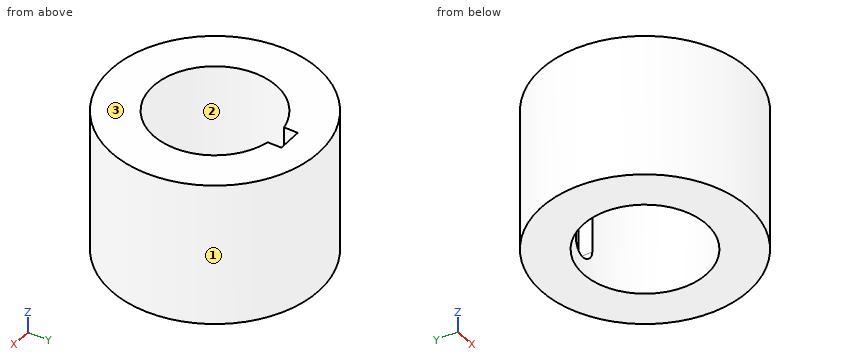
```python
from build123d import *

# Parameters (mm, degrees)
SKETCH1_R           = 21
SKETCH1_R_2         = 12.5
BOSS_EXTRUDE4_DEPTH = 29
SKETCH3_W           = 5
SKETCH3_H           = 5
CUT_EXTRUDE3_DEPTH  = 25.5
FILLET5_R           = 2.5
FILLET6_R           = 2.5


with BuildPart() as part:
    # Sketch1 → Boss-Extrude4 (new body)
    with BuildSketch(Plane.XY):
        with Locations(Location((0, 0, 0), (0, 0, 180))):
            Circle(SKETCH1_R)
        with Locations(Location((0, 0, 0), (0, 0, 180))):
            Circle(SKETCH1_R_2, mode=Mode.SUBTRACT)
    extrude(amount=BOSS_EXTRUDE4_DEPTH)

    # Sketch3 → Cut-Extrude3 (cut)
    with BuildSketch(Plane.XY.offset(29)):
        with Locations((0, 12.5)):
            Rectangle(SKETCH3_W, SKETCH3_H)
    extrude(amount=-CUT_EXTRUDE3_DEPTH, mode=Mode.SUBTRACT)

    # Fillet5
    fillet5_edges = [part.edges().sort_by_distance(p)[0] for p in [
        (2.5, 13.623724357, 3.5),
    ]]
    fillet(fillet5_edges, radius=FILLET5_R)

    # Fillet6
    fillet6_edges = [part.edges().sort_by_distance(p)[0] for p in [
        (-2.5, 13.623724357, 3.5),
    ]]
    fillet(fillet6_edges, radius=FILLET6_R - 0.0001)  # a hair under: the kernel refuses the full size


solid = part.part
```
Can you work these out from the model? Positions are in its coordinate system, mm. Face numbers are marked on the shaded views. Round coordinates to 2 decimals unless told otherwise and drop trailing zeros. Loops run counter-clockwise (first coordinate to the right, second up) from the corner with the lowest first, then second, coordinate; pieces in that order, holes last. Notation, with made-up numbers: (66, -15) -> (107, -15) arc R19 ccw to (107, 21) -> close; hole circle Ø1 at (4, -21). An arc over 180 degrees is marked (long way). One line per item, written item: value. Start each with the question number.
1. If I drill on probe 1 along Y at (x, z) = (0, 22.75); probe 2 along X at (y, z) = (10.5, 7); probe 3 along Y at (x, z) = (4, 26.25), over which ranges is the centre line in solid material (lowest first)?
2. If we section it at D-D, the plane y = -18: Write out the boundary of the cut face in (x, z).
3. If we mould it in two halves opening along X, with no side actions, what happens to the marked faces 1, 2 and 3? For each: pulls with the +X half, pulls with the -X half, needs draft (parallel to the pull), parting line crosses it, or undercut.
4. For pin 1 (1 mm diameter, centred on x = -13.5, z = 6, fed in from +Y); pin 2 (0.8 mm diameter, centred on y = 14.5, z = 21, fed in from -X); pin 3 (5 mm diameter, centred on x = -10, z = 22.5, fed in from +Y), each with a flat end and sliding along its axis, tell me the tip position at first contact or that it passes through.
5. If we section it at C-C, the plane z = 9.5: Write out the boundary of the cut face in (x, y).
6. If we section it at A-A, the plane y = 0: Write out the boundary of the cut face in (x, z).
7. If we section it at B-B, the plane x = 4: Write out the boundary of the cut face in (y, z).
Calculated:
1. probe 1: y = -21 to -12.5, 15 to 21
1. probe 2: x = -18.19 to -6.78, 6.78 to 18.19
1. probe 3: y = -20.62 to -11.84, 11.84 to 20.62
2. outline: (-10.82, 0) -> (10.82, 0) -> (10.82, 29) -> (-10.82, 29) -> close
3. face 1: parting line crosses it
3. face 2: undercut
3. face 3: needs draft
4. pin 1: stops at y = 16.49
4. pin 2: stops at x = -15.56
4. pin 3: stops at y = 19.62
5. outline: circle Ø42 at (0, 0); hole (-2.5, 12.25) arc R12.5 ccw (long way) to (2.5, 12.25) -> (2.5, 15) -> (-2.5, 15) -> close
6. outline: (-21, 0) -> (-12.5, 0) -> (-12.5, 29) -> (-21, 29) -> close; (12.5, 0) -> (21, 0) -> (21, 29) -> (12.5, 29) -> close
7. outline: (-20.62, 0) -> (-11.84, 0) -> (-11.84, 29) -> (-20.62, 29) -> close; (11.84, 0) -> (20.62, 0) -> (20.62, 29) -> (11.84, 29) -> close
